from build123d import *

# Parameters (mm, degrees)
SKETCH1_R             = 85
BOSS_EXTRUDE1_DEPTH   = 7
SKETCH2_R             = 32.5
CUT_EXTRUDE1_DEPTH    = 121.411793442
SKETCH3_R             = 1.625700543
CUT_EXTRUDE2_DEPTH    = 6.872683
CIRPATTERN1_START     = 0.127316845
CIRPATTERN1_OUTLINE_R = 1.625700543
CIRPATTERN1_DEPTH     = 6.872683155


# Read off the part's stored shape, not the designer's step: CirPattern1
with BuildPart() as part:
    # Sketch1 → Boss-Extrude1 (new body)
    with BuildSketch(Plane(origin=(0, 0, 0), x_dir=(1, 0, 0), z_dir=(0, 1, 0))):
        with Locations(Location((0, 0, 0), (0, 0, 270))):
            Circle(SKETCH1_R)
    extrude(amount=BOSS_EXTRUDE1_DEPTH)

    # Sketch2 → Cut-Extrude1 (cut, through all)
    with BuildSketch(Plane(origin=(0, 0, 0), x_dir=(1, 0, 0), z_dir=(0, 1, 0))):
        with Locations(Location((0, 0, 0), (0, 0, 270))):
            Circle(SKETCH2_R)
    extrude(amount=CUT_EXTRUDE1_DEPTH, mode=Mode.SUBTRACT)

    # Sketch3 → Cut-Extrude2 (cut)
    with BuildSketch(Plane(origin=(0, 7, 0), x_dir=(1, 0, 0), z_dir=(0, 1, 0))):
        with Locations(Location((-34.619906271, 0, 0), (0, 0, 270))):
            Circle(SKETCH3_R)
    extrude(amount=-CUT_EXTRUDE2_DEPTH, mode=Mode.SUBTRACT)

    # CirPattern1 outline → CirPattern1 (cut)
    with BuildSketch(Plane(origin=(0, 0, 0), x_dir=(1, 0, 0), z_dir=(0, 1, 0)).offset(CIRPATTERN1_START)):
        with Locations((0, 34.619906271)):
            Circle(CIRPATTERN1_OUTLINE_R)
        with Locations((34.619906271, 0)):
            Circle(CIRPATTERN1_OUTLINE_R)
        with Locations((0, -34.619906271)):
            Circle(CIRPATTERN1_OUTLINE_R)
    extrude(amount=CIRPATTERN1_DEPTH, mode=Mode.SUBTRACT)


solid = part.part
Can you work these out from the model? Positions are in its coordinate system, mm. Round coordinates to 2 decimals unless told otherwise and drop trailing zeros. Order: outer loops, then holes, each group sorted by start corner. A loop starts at its lowest first (then second) coordinate and runs counter-clockwise, first axis right, second up. Notation, with made-up numbers: (-13.75, 16) -> (8.25, 16) arc R32 cw to (8.25, 53) -> close; hole circle Ø5 at (-22, 58.5). An arc over 180 degrees is marked (long way). Write each question's results on one line, items separated by ' | '. Start each with the question number.
Item 1: Please list where these lines run through material, in increasing order: L1, parallel to X at y = 2.75, z = 0; L2, parallel to X at y = 0.75, z = -28.5; L3, parallel to Z at x = 3, y = 3.5.
Item 2: If we section it at C-C, the plane z = -68: Write out the boundary of the cut face in (x, y).
Item 3: Thinking about a two-plate mould opening in X: for faces 1 (the cylindrical face through (-51.721, 3.451, -67.453)), 2 (the cylindrical face through (9.76, 3.45, 31)), 3 (the flat face through (-37, 7, -1)), which applies, +X half, -X half, draft (parallel to the pull), parting line (faces both ways), or undercut?
Item 4: If we section it at B-B, the plane x = 26: Write out the boundary of the cut face in (y, z), then the cut area to 3 significant figures.
Item 5: If we section it at A-A, the plane z = 18: Write out the boundary of the cut face in (x, y), then the cut area to 3 significant figures.
Item 6: Will these pins go through, and if not, where does the flat tip stop? pin 1 (1 mm diameter, centred on x = 0.5, z = -35, fed in from +Y); pin 2 (3 mm diameter, centred on y = 6, z = 55.5, fed in from -X); pin 3 (4 mm diameter, centred on y = 0.5, z = -44.5, fed in from -X).
Item 7: If we section it at D-D, the plane y = 1.25: Write out the boundary of the cut face in (x, z).
Results:
1) L1: x = -85 to -36.25, -32.99 to -32.5, 32.5 to 32.99, 36.25 to 85 | L2: x = -80.08 to -15.62, 15.62 to 80.08 | L3: z = -84.95 to -32.36, 32.36 to 84.95
2) outline: (-51, 0) -> (51, 0) -> (51, 7) -> (-51, 7) -> close
3) face 1: parting line | face 2: undercut | face 3: draft
4) outline: (0, -80.93) -> (7, -80.93) -> (7, -19.5) -> (0, -19.5) -> close; (0, 19.5) -> (7, 19.5) -> (7, 80.93) -> (0, 80.93) -> close | area: 860 mm2
5) outline: (-83.07, 0) -> (-27.06, 0) -> (-27.06, 7) -> (-83.07, 7) -> close; (27.06, 0) -> (83.07, 0) -> (83.07, 7) -> (27.06, 7) -> close | area: 784 mm2
6) pin 1: stops at y = 0.13 | pin 2: stops at x = -65.64 | pin 3: stops at x = -73.61
7) outline: circle Ø170 at (0, 0); hole circle Ø3.25 at (-34.62, 0); hole circle Ø65 at (0, 0); hole circle Ø3.25 at (0, -34.62); hole circle Ø3.25 at (0, 34.62); hole circle Ø3.25 at (34.62, 0)
